```python
from build123d import *

# Parameters (mm, degrees)
BOSS_EXTRUDE1_DEPTH = 4
SKETCH2_R           = 2
SKETCH2_W           = 10
SKETCH2_H           = 80
SKETCH2_W_2         = 35
SKETCH2_H_2         = 80.000000001
CUT_EXTRUDE1_DEPTH  = 10
SKETCH6_R           = 2.5
CUT_EXTRUDE5_DEPTH  = 10
SKETCH11_R          = 2
CUT_EXTRUDE9_DEPTH  = 10
SKETCH16_W          = 40
SKETCH16_H          = 26
CUT_EXTRUDE10_DEPTH = 10
SKETCH17_R          = 2.15
CUT_EXTRUDE11_DEPTH = 10
SKETCH26_R          = 2
CUT_EXTRUDE18_DEPTH = 10
SKETCH28_R          = 4
SKETCH28_R_2        = 2.15
BOSS_EXTRUDE2_DEPTH = 4
SKETCH29_W          = 8
SKETCH29_H          = 4
SKETCH29_W_2        = 29.8
SKETCH29_W_3        = 10
CUT_EXTRUDE19_DEPTH = 10
SKETCH30_R          = 2
CUT_EXTRUDE20_DEPTH = 10


with BuildPart() as part:
    # Sketch1 → Boss-Extrude1 (new body)
    with BuildSketch(Plane.XY):
        with BuildLine():
            Line((-123, 77), (123, 77))
            ThreePointArc((123, 77), (124.414213562, 76.414213562), (125, 75))
            Line((125, 75), (125, -72))
            ThreePointArc((125, -72), (124.414213562, -73.414213562), (123, -74))
            Line((123, -74), (-123, -74))
            ThreePointArc((-123, -74), (-124.414213562, -73.414213562), (-125, -72))
            Line((-125, -72), (-125, 75))
            ThreePointArc((-125, 75), (-124.414213562, 76.414213562), (-123, 77))
        make_face()
    extrude(amount=BOSS_EXTRUDE1_DEPTH)

    # Sketch2 → Cut-Extrude1 (cut)
    with BuildSketch(Plane(origin=(0, 0, 0), x_dir=(-1, 0, 0), z_dir=(0, 0, -1))):
        with Locations((-6.6, -17.5)):
            Circle(SKETCH2_R)
        with Locations((-6.6, 17.5)):
            Circle(SKETCH2_R)
        with Locations((-40, -17.5)):
            Circle(SKETCH2_R)
        with Locations((-40, 17.5)):
            Circle(SKETCH2_R)
        with Locations((6.6, 17.5)):
            Circle(SKETCH2_R)
        with Locations((6.6, -17.5)):
            Circle(SKETCH2_R)
        with Locations((40, -17.5)):
            Circle(SKETCH2_R)
        with Locations((40, 17.5)):
            Circle(SKETCH2_R)
        with Locations((-120, 0)):
            Rectangle(SKETCH2_W, SKETCH2_H)
        with Locations((-62.5, -1e-09)):
            Rectangle(SKETCH2_W_2, SKETCH2_H_2)
        with Locations((120, 0)):
            Rectangle(SKETCH2_W, SKETCH2_H)
        with Locations((62.5, -1e-09)):
            Rectangle(SKETCH2_W_2, SKETCH2_H_2)
    extrude(amount=-CUT_EXTRUDE1_DEPTH, mode=Mode.SUBTRACT)

    # Sketch6 → Cut-Extrude5 (cut)
    with BuildSketch(Plane(origin=(0, 0, 0), x_dir=(-1, 0, 0), z_dir=(0, 0, -1))):
        with Locations((-104, -25.5)):
            Circle(SKETCH6_R)
        with Locations((-104, 25.5)):
            Circle(SKETCH6_R)
        with Locations((104, -25.5)):
            Circle(SKETCH6_R)
        with Locations((104, 25.5)):
            Circle(SKETCH6_R)
    extrude(amount=-CUT_EXTRUDE5_DEPTH, mode=Mode.SUBTRACT)

    # Sketch11 → Cut-Extrude9 (cut)
    with BuildSketch(Plane(origin=(0, 0, 0), x_dir=(-1, 0, 0), z_dir=(0, 0, -1))):
        with Locations((-17, -62.5)):
            Circle(SKETCH11_R)
        with Locations((17, -62.5)):
            Circle(SKETCH11_R)
        with Locations((-17, 65.5)):
            Circle(SKETCH11_R)
        with Locations((17, 65.5)):
            Circle(SKETCH11_R)
        with BuildLine():
            Line((-9, -54), (9, -54))
            ThreePointArc((9, -54), (11.121320344, -54.878679656), (12, -57))
            Line((12, -57), (12, -68))
            ThreePointArc((12, -68), (11.121320344, -70.121320344), (9, -71))
            Line((9, -71), (-9, -71))
            ThreePointArc((-9, -71), (-11.121320344, -70.121320344), (-12, -68))
            Line((-12, -68), (-12, -57))
            ThreePointArc((-12, -57), (-11.121320344, -54.878679656), (-9, -54))
        make_face()
        with BuildLine():
            Line((-9, 74), (9, 74))
            ThreePointArc((9, 74), (11.121320344, 73.121320344), (12, 71))
            Line((12, 71), (12, 60))
            ThreePointArc((12, 60), (11.121320344, 57.878679656), (9, 57))
            Line((9, 57), (-9, 57))
            ThreePointArc((-9, 57), (-11.121320344, 57.878679656), (-12, 60))
            Line((-12, 60), (-12, 71))
            ThreePointArc((-12, 71), (-11.121320344, 73.121320344), (-9, 74))
        make_face()
    extrude(amount=-CUT_EXTRUDE9_DEPTH, mode=Mode.SUBTRACT)

    # Sketch16 → Cut-Extrude10 (cut)
    with BuildSketch(Plane(origin=(0, 0, 0), x_dir=(-1, 0, 0), z_dir=(0, 0, -1))):
        with Locations((-93, 64)):
            Rectangle(SKETCH16_W, SKETCH16_H)
        with Locations((93, 64)):
            Rectangle(SKETCH16_W, SKETCH16_H)
    extrude(amount=-CUT_EXTRUDE10_DEPTH, mode=Mode.SUBTRACT)

    # Sketch17 → Cut-Extrude11 (cut)
    with BuildSketch(Plane(origin=(0, 0, 0), x_dir=(-1, 0, 0), z_dir=(0, 0, -1))):
        with Locations((67.6, 65.6)):
            Circle(SKETCH17_R)
        with Locations((67.6, 55.4)):
            Circle(SKETCH17_R)
        with Locations((115.4, 55.4)):
            Circle(SKETCH17_R)
        with Locations((115.4, 65.6)):
            Circle(SKETCH17_R)
        with Locations((-115.4, 65.6)):
            Circle(SKETCH17_R)
        with Locations((-115.4, 55.4)):
            Circle(SKETCH17_R)
        with Locations((-67.6, 55.4)):
            Circle(SKETCH17_R)
        with Locations((-67.6, 65.6)):
            Circle(SKETCH17_R)
    extrude(amount=-CUT_EXTRUDE11_DEPTH, mode=Mode.SUBTRACT)

    # Sketch26 → Cut-Extrude18 (cut)
    with BuildSketch(Plane(origin=(0, 0, 0), x_dir=(-1, 0, 0), z_dir=(0, 0, -1))):
        with Locations((-112, -51)):
            Circle(SKETCH26_R)
        with Locations((-65, -51)):
            Circle(SKETCH26_R)
        with Locations((65, -51)):
            Circle(SKETCH26_R)
        with Locations((112, -51)):
            Circle(SKETCH26_R)
    extrude(amount=-CUT_EXTRUDE18_DEPTH, mode=Mode.SUBTRACT)

    # Sketch28 → Boss-Extrude2 (add)
    # profile 1 of 4: a face of its own
    with BuildSketch(Plane(origin=(0, 0, 0), x_dir=(-1, 0, 0), z_dir=(0, 0, -1))):
        with Locations((-115.4, 65.6)):
            Circle(SKETCH28_R)
        with Locations((-115.4, 65.6)):
            Circle(SKETCH28_R_2, mode=Mode.SUBTRACT)
    # profile 2 of 4: a face of its own
    with BuildSketch(Plane(origin=(0, 0, 0), x_dir=(-1, 0, 0), z_dir=(0, 0, -1))):
        with Locations((-115.4, 55.4)):
            Circle(SKETCH28_R)
        with Locations((-115.4, 55.4)):
            Circle(SKETCH28_R_2, mode=Mode.SUBTRACT)
    # profile 3 of 4: a face of its own
    with BuildSketch(Plane(origin=(0, 0, 0), x_dir=(-1, 0, 0), z_dir=(0, 0, -1))):
        with Locations((115.4, 55.4)):
            Circle(SKETCH28_R)
        with Locations((115.4, 55.4)):
            Circle(SKETCH28_R_2, mode=Mode.SUBTRACT)
    # profile 4 of 4: a face of its own
    with BuildSketch(Plane(origin=(0, 0, 0), x_dir=(-1, 0, 0), z_dir=(0, 0, -1))):
        with Locations((115.4, 65.6)):
            Circle(SKETCH28_R)
        with Locations((115.4, 65.6)):
            Circle(SKETCH28_R_2, mode=Mode.SUBTRACT)
    extrude(amount=-BOSS_EXTRUDE2_DEPTH)

    # Sketch29 → Cut-Extrude19 (cut)
    with BuildSketch(Plane.XY.offset(4)):
        with Locations((-31, -52)):
            Rectangle(SKETCH29_W, SKETCH29_H)
        with Locations((31, -52)):
            Rectangle(SKETCH29_W, SKETCH29_H)
        with Locations((0.1, -37)):
            Rectangle(SKETCH29_W_2, SKETCH29_H)
        with Locations((0.1, 37)):
            Rectangle(SKETCH29_W_2, SKETCH29_H)
        with Locations((32.15, 69)):
            Rectangle(SKETCH29_W_3, SKETCH29_H)
        with Locations((-32.15, 69)):
            Rectangle(SKETCH29_W_3, SKETCH29_H)
    extrude(amount=-CUT_EXTRUDE19_DEPTH, mode=Mode.SUBTRACT)

    # Sketch30 → Cut-Extrude20 (cut)
    with BuildSketch(Plane(origin=(0, 0, 0), x_dir=(-1, 0, 0), z_dir=(0, 0, -1))):
        with Locations((43.4, 69)):
            Circle(SKETCH30_R)
        with Locations((-43.4, 69)):
            Circle(SKETCH30_R)
        with Locations((-29.39999999, 37)):
            Circle(SKETCH30_R)
        with Locations((29.39999999, 37)):
            Circle(SKETCH30_R)
        with Locations((29.39999999, -37)):
            Circle(SKETCH30_R)
        with Locations((-29.39999999, -37)):
            Circle(SKETCH30_R)
        with Locations((-43, -52)):
            Circle(SKETCH30_R)
        with Locations((43, -52)):
            Circle(SKETCH30_R)
    extrude(amount=-CUT_EXTRUDE20_DEPTH, mode=Mode.SUBTRACT)


solid = part.part
```
Source: CAD feature listing. Evaluate the final solid. Frame: model axes, mm. Give positions to 0.01 mm unless a question says otherwise; leave off trailing zeros. Write each loop counter-clockwise with the first axis right and the second up, starting at its lowest first coordinate (ties: lowest second). Pieces come first, ordered by that corner, then holes.
1. Section query B-B (z = 0.9). Count the separate pieces of the cut face and the enclosed holes in it, then the cut area to 3 significant figures.
2. First-contact query: pin 1 (2 mm diameter, centred on x = -88, z = 2.5, fed in from +Y); pin 2 (2 mm diameter, centred on y = 12, z = 2, fed in from +X). Flat tips, straight axial feed; report the tip coordinate or a pass-through.
3. Section query A-A (x = 56.5). Return the cut outline in (y, z), then the cut area to 3 significant figures.
4. Pull-direction query (X, two-part tool) for faces 1 (the face through (2, -14, 0)), 2 (the face through (-106.385, -24.749, 1.972)); classes: +X half, -X half, draft (parallel to the pull), parting line (faces both ways), or undercut.
5. Material intervals for line 1 along X through (y, z) = (-34, 2.85); line 2 along Y through (x, z) = (40, 2.9); line 3 along Y through (x, z) = (-43, 2.1), sorted ascending.
Output values:
1. separate pieces: 1
1. enclosed holes: 46
1. area: 26,800 mm2
2. pin 1: stops at y = 51
2. pin 2: stops at x = 115
3. outline: (-74, 0) - (-40, 0) - (-40, 4) - (-74, 4) - close; (40, 0) - (77, 0) - (77, 4) - (40, 4) - close
3. area: 284 mm2
4. face 1: draft
4. face 2: undercut
5. line 1: x = -115 to -80, -45 to 45, 80 to 115
5. line 2: y = -74 to -19.5, -15.5 to 15.5, 19.5 to 77
5. line 3: y = -74 to -54, -50 to 67.04, 70.96 to 77
